Design review of the part built by this model. Coordinates are the model's own, in mm. Give positions to 0.01 mm unless a question says otherwise; leave off trailing zeros. One line per item, written item: value.
from build123d import *

# Parameters (mm, degrees)
SKETCH1_R                   = 107.95
SKETCH1_R_2                 = 96.8375
BOSS_EXTRUDE1_DEPTH         = 3.175
SKETCH2_R                   = 2.38125
BOSS_EXTRUDE2_START         = -6.35
BOSS_EXTRUDE2_DEPTH         = 6.35
BOSS_EXTRUDE3_START         = -6.35
SKETCH7_R                   = 14.2875
BOSS_EXTRUDE3_DEPTH         = 6.35
FILLET1_R                   = 7.62
CIRPATTERN1_START           = -3.175
CIRPATTERN1_DEPTH           = 6.35
F_1_4_CLEARANCE_HOLE1_D     = 6.7564
F_1_4_CLEARANCE_HOLE1_DEPTH = 9.398
F_1_4_CLEARANCE_HOLE1_TIP   = 2.029827343
FILLET2_R                   = 7.62


# Read off the part's stored shape, not the designer's step: CirPattern1
with BuildPart() as part:
    # Sketch1 → Boss-Extrude1 (new, symmetric)
    with BuildSketch(Plane(origin=(0, 0, 0), x_dir=(1, 0, 0), z_dir=(0, 1, 0))):
        with Locations(Location((0, 0, 0), (0, 0, 270))):
            Circle(SKETCH1_R)
        with Locations(Location((0, 0, 0), (0, 0, 270))):
            Circle(SKETCH1_R_2, mode=Mode.SUBTRACT)
    extrude(amount=BOSS_EXTRUDE1_DEPTH, both=True)

    # Sketch2 → Cut-Revolve1 (revolve, cut)
    with BuildSketch(Plane(origin=(0, 0, 0), x_dir=(0, 0, -1), z_dir=(1, 0, 0)), mode=Mode.PRIVATE) as cut_revolve1_sk:
        with Locations((-101.6, -4.445)):
            Circle(SKETCH2_R)
    revolve(cut_revolve1_sk.sketch.rotate(Axis((0, -31.187956177, 0), (0, 1, 0)), 180), axis=Axis((0, -31.187956177, 0), (0, 1, 0)), mode=Mode.SUBTRACT)

    # Sketch3 → Boss-Extrude2 (add)
    with BuildSketch(Plane(origin=(0, 3.175, 0), x_dir=(1, 0, 0), z_dir=(0, 1, 0)).offset(BOSS_EXTRUDE2_START)):
        with BuildLine():
            Line((-5.499261314, -82.55), (-13.224366326, -95.930274374))
            ThreePointArc((-13.224366326, -95.930274374), (0, -96.8375), (13.224366326, -95.930274374))
            Line((13.224366326, -95.930274374), (5.499261314, -82.55))
            ThreePointArc((5.499261314, -82.55), (0, -79.375), (-5.499261314, -82.55))
        make_face()
    extrude(amount=BOSS_EXTRUDE2_DEPTH)

    # Sketch7 → Boss-Extrude3 (add)
    with BuildSketch(Plane(origin=(0, 3.175, 0), x_dir=(1, 0, 0), z_dir=(0, 1, 0)).offset(BOSS_EXTRUDE3_START)):
        with BuildLine():
            ThreePointArc((76.789392316, 58.999073162), (48.41875, 83.863735039), (12.7, 96.001101068))
            Line((12.7, 96.001101068), (12.7, 60.491874454))
            ThreePointArc((12.7, 60.491874454), (23.8125, 41.244459855), (46.0375, 41.244459855))
            Line((46.0375, 41.244459855), (76.789392316, 58.999073162))
        make_face()
        with Locations(Location((34.925, 60.491874454, 0), (0, 0, 270))):
            Circle(SKETCH7_R, mode=Mode.SUBTRACT)
    extrude(amount=BOSS_EXTRUDE3_DEPTH)

    # Fillet1
    fillet1_edges = [part.edges().sort_by_distance(p)[0] for p in [
        (-13.224366326, 0, 95.930274374),
        (13.224366326, 0, 95.930274374),
    ]]
    fillet(fillet1_edges, radius=FILLET1_R)

    # CirPattern1 outline → CirPattern1 (add)
    with BuildSketch(Plane(origin=(0, 0, 0), x_dir=(1, 0, 0), z_dir=(0, 1, 0)).offset(CIRPATTERN1_START)):
        with BuildLine():
            ThreePointArc((72.968215537, -63.664282982), (83.863735039, -48.41875), (91.618994144, -31.360186833))
            ThreePointArc((91.618994144, -31.360186833), (88.840241596, -35.092023113), (84.409630671, -36.5125))
            Line((84.409630671, -36.5125), (74.240027739, -36.5125))
            ThreePointArc((74.240027739, -36.5125), (68.740766425, -39.6875), (68.740766425, -46.0375))
            Line((68.740766425, -46.0375), (73.825567891, -54.844634485))
            ThreePointArc((73.825567891, -54.844634485), (74.810704284, -59.391894543), (72.968215537, -63.664282982))
        make_face()
        with BuildLine():
            Line((75.941505111, 58.509545256), (68.740766425, 46.0375))
            ThreePointArc((68.740766425, 46.0375), (68.740766425, 39.6875), (74.240027739, 36.5125))
            Line((74.240027739, 36.5125), (84.409630671, 36.5125))
            ThreePointArc((84.409630671, 36.5125), (88.840241596, 35.092023113), (91.618994145, 31.360186833))
            ThreePointArc((91.618994145, 31.360186833), (85.330669556, 45.784039133), (76.789392316, 58.999073162))
            Line((76.789392316, 58.999073162), (75.941505111, 58.509545256))
        make_face()
        with BuildLine():
            ThreePointArc((-84.409630671, -36.5125), (-88.840241596, -35.092023113), (-91.618994145, -31.360186833))
            ThreePointArc((-91.618994145, -31.360186833), (-83.863735039, -48.41875), (-72.968215537, -63.664282982))
            ThreePointArc((-72.968215537, -63.664282982), (-74.810704284, -59.391894543), (-73.825567891, -54.844634485))
            Line((-73.825567891, -54.844634485), (-68.740766425, -46.0375))
            ThreePointArc((-68.740766425, -46.0375), (-68.740766425, -39.6875), (-74.240027739, -36.5125))
            Line((-74.240027739, -36.5125), (-84.409630671, -36.5125))
        make_face()
        with BuildLine():
            ThreePointArc((12.7, 96.001101068), (-3.015193802, 96.790547124), (-18.650778608, 95.024469815))
            ThreePointArc((-18.650778608, 95.024469815), (-14.029537312, 94.483917657), (-10.58406278, 91.357134485))
            Line((-10.58406278, 91.357134485), (-5.499261314, 82.55))
            ThreePointArc((-5.499261314, 82.55), (0, 79.375), (5.499261314, 82.55))
            Line((5.499261314, 82.55), (12.7, 95.022045256))
            Line((12.7, 95.022045256), (12.7, 96.001101068))
        make_face()
        with BuildLine():
            Line((-68.740766425, 46.0375), (-73.825567891, 54.844634485))
            ThreePointArc((-73.825567891, 54.844634485), (-74.810704284, 59.391894543), (-72.968215537, 63.664282982))
            ThreePointArc((-72.968215537, 63.664282982), (-83.863735039, 48.41875), (-91.618994145, 31.360186833))
            ThreePointArc((-91.618994145, 31.360186833), (-88.840241596, 35.092023113), (-84.409630671, 36.5125))
            Line((-84.409630671, 36.5125), (-74.240027739, 36.5125))
            ThreePointArc((-74.240027739, 36.5125), (-68.740766425, 39.6875), (-68.740766425, 46.0375))
        make_face()
    extrude(amount=CIRPATTERN1_DEPTH)

    # 1/4 Clearance Hole1
    with Locations(Plane(origin=(0, 3.175, 0), x_dir=(1, 0, 0), z_dir=(0, 1, 0))):
        with Locations((0, -85.725), (74.240027739, -42.8625), (74.240027739, 42.8625), (-74.240027739, 42.8625), (-74.240027739, -42.8625), (0, 85.725)):
            Hole(F_1_4_CLEARANCE_HOLE1_D / 2, depth=F_1_4_CLEARANCE_HOLE1_DEPTH)
            with Locations((0, 0, -(F_1_4_CLEARANCE_HOLE1_DEPTH + F_1_4_CLEARANCE_HOLE1_TIP / 2))):  # 118° drill point
                Cone(0, F_1_4_CLEARANCE_HOLE1_D / 2, F_1_4_CLEARANCE_HOLE1_TIP, mode=Mode.SUBTRACT)

    # Fillet2
    fillet2_edges = [part.edges().sort_by_distance(p)[0] for p in [
        (75.941505111, 0, -58.509545256),
        (12.7, 0, -95.022045256),
    ]]
    fillet(fillet2_edges, radius=FILLET2_R)


solid = part.part
Item 1: Add section B-B on y = 0.5. Count the separate pieces of the cut face and the enclosed holes in it, plus the area to 3 significant figures.
Returned:
separate pieces: 1
enclosed holes: 8
area: 10,600 mm²
Item 2: Clearance check with flat-ended pins moving along their axes: P1, Ø2, axis at x = -72.5, y = 2, coming from the -Z side; P2, Ø3, axis at x = -80, y = 0.5, coming from the -Z side; P3, Ø3, axis at x = -80.5, y = -1, coming from the +Z side. State where each tip first meets the part, or that it passes through.
Returned:
P1: z = -80.88
P2: z = -74.1
P3: z = 73.57
Item 3: Draft analysis for pull direction X (two halves, no side actions). For faces 1 (the flat face through (22, -3.175, -45)), 2 (the cylindrical face through (23.53, -0.04, -41.41)), state which applies: pulls with the +X half, pulls with the -X half, needs draft (parallel to the pull), parting line crosses it, or undercut.
Returned:
face 1: needs draft
face 2: undercut
Item 4: To check wall thickness, follow line 1 along X through (y, z) = (1.75, -66); line 2 along X through (y, z) = (1.25, -84); line 3 along X through (y, z) = (-0.25, -3). State the ranges of each line that lie inside material, in increasing order. Write a range as from..to.
Returned:
line 1: -85.42..-70.86, 12.7..21.74, 48.11..85.42
line 2: -67.8..-48.18, -6.34..-2.9, 2.9..67.8
line 3: -107.91..-96.79, 96.79..107.91
